Verification items for the finished model (mm, model axes). A direction names the side the tool comes from. Give positions to 0.01 mm unless a question says otherwise; leave off trailing zeros. Order: outer loops, then holes, each group sorted by start corner. A loop starts at its lowest first (then second) coordinate and runs counter-clockwise, first axis right, second up. Notation, with made-up numbers: (44.25, 8.25) - (55.25, 8.25) arc R7 ccw to (55.25, 14.25) - close; hole circle Ø8 at (-22.5, 30). An arc over 180 degrees is marked (long way). Answer as a JSON object with one key per item and string values.
Autodesk Inventor part; units mm, degrees
ref_plane "YZ Plane" through (0, 0, 0) normal (1, 0, 0) x (0, 1, 0)
ref_plane "XZ Plane" through (0, 0, 0) normal (0, 1, 0) x (-1, 0, 0)
ref_plane "XY Plane" through (0, 0, 0) normal (0, 0, 1) x (1, 0, 0)
sketch "Sketch1" plane through (0, 0, 0) normal (0, 0, 1) x (1, 0, 0)
  line L0 (0, 0) -> (110, 0)
  line L1 (110, 0) -> (110, 50)
  line L2 (110, 50) -> (0, 50)
  line L3 (0, 50) -> (0, 0)
  circle A0 centre (80, 25) radius 4
  circle A1 centre (30, 25) radius 4
  line L4 (30, 25) -> (80, 25) construction
  point P0 (110, 25)
  dimension "d0" = 110
  dimension "d1" = 50
  dimension "d2" = 8
  dimension "d3" = 8
  dimension "d4" = 50
  dimension "d5" = 30
extrude "Extrusion1" add sketch "Sketch1" along normal blind 10
sketch "Sketch2" plane through (0, 50, 0) normal (0, 1, 0) x (1, 0, 0)
  line L0 (110, -10) -> (0, -10)
  line L1 (0, -10) -> (110, -10)
  line L2 (110, -10) -> (110, 28.1)
  line L3 (110, 28.1) -> (0, 28.1)
  line L4 (0, 28.1) -> (0, -10)
  point P0 (0, 0)
  dimension "d8" = 38.1
extrude "Extrusion2" add sketch "Sketch2" against normal blind 10
properties part number "BA03"
(1) Section check D-D (x = 40). Record the cut outline in (y, z).
Computed values:
{"outline": "(0, 0) - (40, 0) - (40, -28.1) - (50, -28.1) - (50, 10) - (0, 10) - close"}
(2) Section check C-C (z = 6.5). Record the cut outline in (x, y), then the cut area to 3 significant figures.
Computed values:
{"outline": "(0, 0) - (110, 0) - (110, 50) - (0, 50) - close; hole circle Ø8 at (30, 25); hole circle Ø8 at (80, 25)", "area": "5,400 mm²"}
(3) Gauge pin test, flat end, axial feed: pin 1 Ø13 at (x, y) = (30, 25) entering from -Z. Record the tip position at first contact, or that the pin passes through.
Computed values:
{"pin 1": "stops at z = 0"}
(4) Access from +Z, -Z, +X, -X, +Y, -Y to the whole of each face (thin tool, end or side, straight path). Record for faces 1 (the flat face through (54, 25, 10)), 2 (the flat face through (54, 20, 0)).
Computed values:
{"face 1": "+Z, +X, -X, +Y, -Y", "face 2": "-Z, +X, -X, -Y"}
(5) Section check B-B (y = 25). Record the cut outline in (x, z).
Computed values:
{"outline": "(0, 0) - (26, 0) - (26, 10) - (0, 10) - close; (34, 0) - (76, 0) - (76, 10) - (34, 10) - close; (84, 0) - (110, 0) - (110, 10) - (84, 10) - close"}
(6) Material ranges on line 1 along Y through (x, z) = (30, 5); line 2 along X through (y, z) = (23.5, 6); line 3 along X through (y, z) = (27, 7.5), recorded low to high. Write a range as [from, to].
Computed values:
{"line 1": "y = [0, 21], [29, 50]", "line 2": "x = [0, 26.29], [33.71, 76.29], [83.71, 110]", "line 3": "x = [0, 26.54], [33.46, 76.54], [83.46, 110]"}
(7) Section check A-A (x = 80). Record the cut outline in (y, z).
Computed values:
{"outline": "(0, 0) - (21, 0) - (21, 10) - (0, 10) - close; (29, 0) - (40, 0) - (40, -28.1) - (50, -28.1) - (50, 10) - (29, 10) - close"}
(8) Release check for a two-part mould opening along Y. For faces 3 (the flat face through (0, 36, 3)), 4 (the flat face through (54, 0, 5)), 5 (the cylindrical face through (77.05, 22.3, 4.93)), 6 (the cylindrical face through (27.05, 22.3, 4.93)) record: pulls with the +Y half, pulls with the -Y half, needs draft (parallel to the pull), parting line crosses it, or undercut.
Computed values:
{"face 3": "needs draft", "face 4": "pulls with the -Y half", "face 5": "undercut", "face 6": "undercut"}
